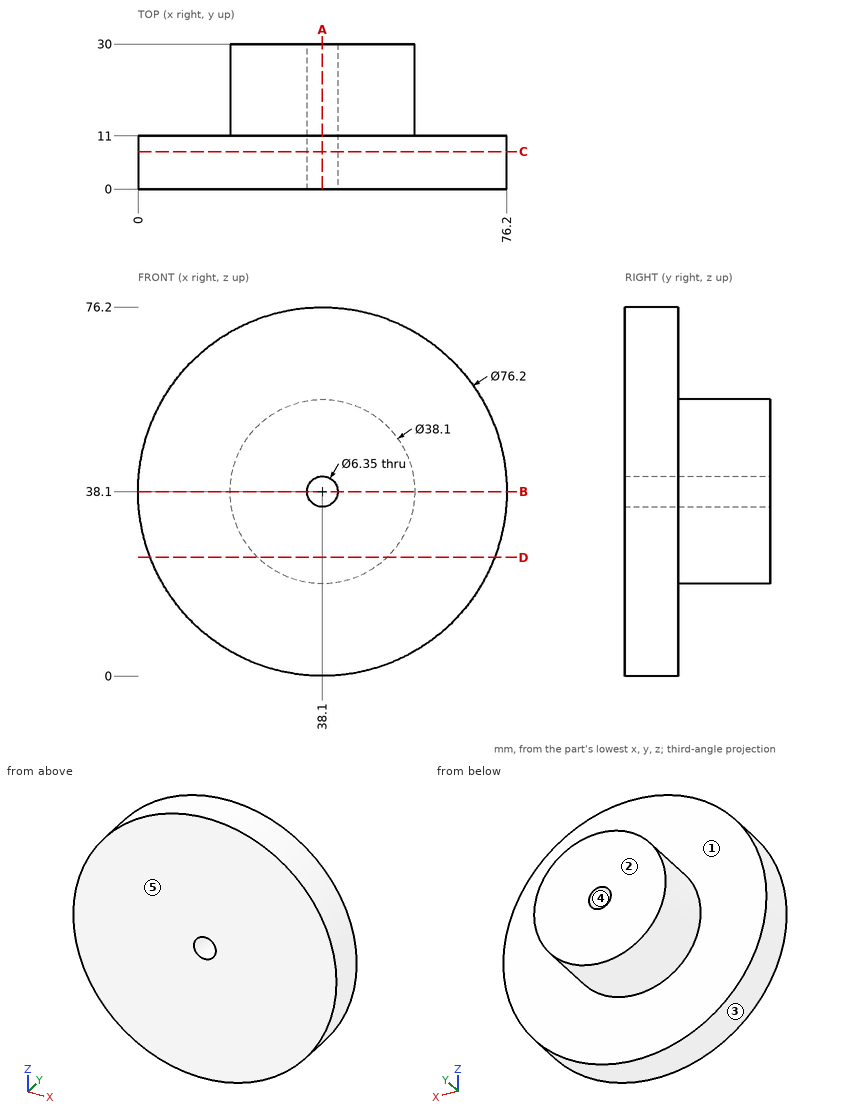
Answer from the drawing. Dimensions are ordinates in mm from the lowest x, y and z of the part. A direction names the side the tool comes from. Give positions to 0.01 mm unless a question says otherwise; leave off trailing zeros. Order: outer loops, then holes, each group sorted by start corner. A loop starts at its lowest first (then second) coordinate and runs counter-clockwise, first axis right, second up. Notation, with made-up numbers: (-29, 45) -> (1, 45) arc R23 cw to (1, 69) -> close; hole circle Ø5 at (-40, 46). An arc over 180 degrees is marked (long way). One line per item, written item: value. Start each with the question number.
(1) A tool of negligible diameter and unlimited length cuts with its end or side. For the marked faces 1 and 2, from which of +Z, -Z, +X, -X, +Y, -Y can it reach the whole face along a straight path? Write none if from no direction.
(2) The part is cut by section B-B (z = 38.1). Determine the outline of the cut face in (x, y) (3 decimals), and give its area (3 significant figures).
(3) For a pull along X with two mould halves and no side action, classify the marked faces 3, 4 and 5 as released by +X, released by -X, zero draft, split by the parting line, or undercut.
(4) Straight lines are drawn through the part: L1, parallel to Z at x = 38.1, y = 6.75 (3 decimals); L2, parallel to Z at x = 38.1, y = 19.5 (3 decimals). For each, find the intervals that lie inside material, in ascending order.
(5) The part is cut by section C-C (y = 7.75). Determine the outline of the cut face in (x, z) (3 decimals), and give its area (3 significant figures).
(6) The part is cut by section A-A (x = 38.1). Determine the outline of the cut face in (y, z) (3 decimals), and give its area (3 significant figures).
(7) Flat-ended cylindrical pins translate along their axes: P1, Ø2, axis at x = 58, z = 55, coming from the -Y side; P2, Ø10, axis at y = 19, z = 26, coming from the -X side; P3, Ø3, axis at x = 9, y = 5, coming from the -Z side (3 decimals); P4, Ø6, axis at y = 7, z = 32, coming from the +X side. Find the tip coordinate at first contact, or state that the pin passes through.
(8) The part is cut by section D-D (z = 24.5). Determine the outline of the cut face in (x, y), and give its area (3 significant figures).
Taken from the geometry:
1. face 1: +Y
1. face 2: +Z, -Z, +X, -X, +Y
2. outline: (0, 0) -> (34.925, 0) -> (34.925, 30) -> (19.05, 30) -> (19.05, 11) -> (0, 11) -> close; (41.275, 0) -> (76.2, 0) -> (76.2, 11) -> (57.15, 11) -> (57.15, 30) -> (41.275, 30) -> close
2. area: 1,370 mm^2
3. face 3: split by the parting line
3. face 4: undercut
3. face 5: zero draft
4. L1: 0 to 34.925, 41.275 to 76.2
4. L2: 19.05 to 34.925, 41.275 to 57.15
5. outline: circle Ø76.2 at (38.1, 38.1); hole circle Ø6.35 at (38.1, 38.1)
5. area: 4,530 mm^2
6. outline: (0, 0) -> (11, 0) -> (11, 19.05) -> (30, 19.05) -> (30, 34.925) -> (0, 34.925) -> close; (0, 41.275) -> (30, 41.275) -> (30, 57.15) -> (11, 57.15) -> (11, 76.2) -> (0, 76.2) -> close
6. area: 1,370 mm^2
7. P1: y = 0
7. P2: x = 20.42
7. P3: z = 11.835
7. P4: x = 76.07
8. outline: (2.51, 0) -> (73.69, 0) -> (73.69, 11) -> (51.44, 11) -> (51.44, 30) -> (24.76, 30) -> (24.76, 11) -> (2.51, 11) -> close
8. area: 1,290 mm^2
